For this review, take the finished solid that the model builds, in its own axes (mm). A direction names the side the tool comes from. Coordinates: 2 decimals unless noted, no trailing zeros. Loops run counter-clockwise (first coordinate to the right, second up) from the corner with the lowest first, then second, coordinate; pieces in that order, holes last. Notation, with made-up numbers: (-16, 7.25) - (-1, 7.25) arc R30 ccw to (-1, 37.25) - close; hole circle Ø3 at (39.25, 4). An arc over 180 degrees is marked (long way). Use one line per item in the form item = value. Start each with the question number.
1. Machinability: for faces 1 (the face through (-15, 1, 2)), 2 (the face through (30.35, 0.49, 38.32)), which of the approach directions +Z, -Z, +X, -X, +Y, -Y give a long, thin tool a straight path to every point of the face, cutting with its end or side? Answer none if there is none.
2. For pin 1 Ø6 at (x, z) = (20, -150) entering from -Y, flat-tipped, find the tip position at first contact; note if it passes through.
3. Add section B-B on z = -8. Give the boundary of the cut face in (x, y), and give its area (3 significant figures).
4. Add section A-A on y = 0.25. Count the separate pieces of the cut face and the enclosed holes in it, and give its area (3 significant figures).
5. Add section C-C on z = 113.5. Give the boundary of the cut face in (x, y).
6. To check wall thickness, follow probe 1 along Z at (x, y) = (-140, 0.75); probe 2 along X at (y, z) = (0.3, -150); probe 3 along X at (y, z) = (0.5, 150). State the ranges of each line that lie inside material, in increasing order.
Autodesk Inventor part; units mm, degrees
ref_plane "YZ Plane" through (0, 0, 0) normal (1, 0, 0) x (0, 1, 0)
ref_plane "XZ Plane" through (0, 0, 0) normal (0, 1, 0) x (-1, 0, 0)
ref_plane "XY Plane" through (0, 0, 0) normal (0, 0, 1) x (1, 0, 0)
sketch "Sketch1" plane through (0, 0, 0) normal (0, 1, 0) x (-1, 0, 0)
  line L0 (150, 160) -> (-190, 160)
  line L1 (-190, 160) -> (-190, -160)
  line L2 (-190, -160) -> (150, -160)
  line L3 (150, -160) -> (150, 160)
  line L4 (-20, -80) -> (0.9973, 160)
  line L5 (-20, -80) -> (220.9168, -80) construction
  line L6 (-20, -80) -> (-40.9973, 160)
  line L7 (140, -150) -> (-180, -150)
  line L8 (-180, -150) -> (-180, 150)
  line L9 (140, 150) -> (140, -150)
  circle A0 centre (140, 150) radius 2.5
  circle A1 centre (-180, 150) radius 2.5
  line L10 (140, 160) -> (140, 50)
  line L11 (140, 50) -> (140, -50)
  circle A2 centre (140, 50) radius 2.5
  circle A3 centre (140, -50) radius 2.5
  circle A4 centre (140, -150) radius 2.5
  circle A5 centre (-180, 50) radius 2.5
  circle A6 centre (-180, -50) radius 2.5
  circle A7 centre (-180, -150) radius 2.5
  circle A8 centre (-20, -150) radius 2.5
  line L12 (150, -150) -> (140, -150)
  line L13 (-20, -150) -> (-20, -80)
  point P0 (0, 0)
  point P1 (-40.9973, 160)
  dimension "d0" = 340
  dimension "d1" = 320
  dimension "d2" = 85
  dimension "d3" = 10
  dimension "d4" = 5
  dimension "d5" = 5
  dimension "d6" = 110
  dimension "d7" = 100
  dimension "d8" = 5
  dimension "d9" = 5
  dimension "d10" = 5
  dimension "d11" = 5
  dimension "d14" = 10
extrude "Extrusion1" add sketch "Sketch1" along normal blind 1 contours L3 L12 A4 L9 A3 A2 A0 L10 L0 | L10 A0 L9 A2 A3 A4 L7 A8 L13 L4 L0 | L3 L2 L1 L0 L6 L13 A8 L7 A4 L12
properties part number "PuertaCuero"
Conclusion:
q1.face_1 = +Z, -Z, +X, -X, +Y
q1.face_2 = +Z, +Y, -Y
q2.pin_1 = 0
q3.outline = (-150, 0) - (13.7, 0) - (13.7, 1) - (-150, 1) - close; (26.3, 0) - (190, 0) - (190, 1) - (26.3, 1) - close
q3.area = 327 mm^2
q4.separate_pieces = 1
q4.enclosed_holes = 9
q4.area = 104,000 mm^2
q5.outline = (-150, 0) - (3.07, 0) - (3.07, 1) - (-150, 1) - close; (36.93, 0) - (190, 0) - (190, 1) - (36.93, 1) - close
q6.probe_1 = -160 to -152.5, -147.5 to -52.5, -47.5 to 47.5, 52.5 to 147.5, 152.5 to 160
q6.probe_2 = -150 to -142.5, -137.5 to 17.5, 22.5 to 177.5, 182.5 to 190
q6.probe_3 = -150 to -142.5, -137.5 to -0.12, 40.12 to 177.5, 182.5 to 190
